Study the drawing (mm; zero at the part's minimum x, y, z) and answer. A direction names the side the tool comes from. Coordinates: 2 decimals unless noted, no trailing zeros. Order: outer loops, then holes, each group sorted by start corner. A loop starts at its lowest first (then second) coordinate and runs counter-clockwise, first axis right, second up. Notation, with made-up numbers: (18.25, 50.5) -> (68.25, 50.5) arc R32 cw to (68.25, 79.5) -> close; hole circle Ø8 at (29, -33.75). An arc over 180 degrees is marked (long way). Answer as CSV lines item,"result". Start each with the question number.
Item 1: Each of these flat-tipped pins is pushed along its axis until it touches: pin 1 Ø1.5 at (y, z) = (3.5, 1) entering from +X; pin 2 Ø2 at (x, z) = (10, 2) entering from +Y. Where does it stop, or does it pass through?
Item 2: Which of the six approach directions +Z, -Z, +X, -X, +Y, -Y give full straight-line access (tool end or side, diameter ignored) to the marked faces 4, 5 and 6?
Item 3: Section B-B (z = 4) is taken. Write down the section's boundary in (x, y), then the cut area to 3 significant figures.
Item 4: For a pull along Y with two mould halves and no side action, classify the marked faces 1, 2 and 3 as pulls with the +Y half, pulls with the -Y half, needs draft (parallel to the pull), parting line crosses it, or undercut.
Item 5: Section A-A (x = 16.3) is taken. Write down the section's boundary in (y, z), then the cut area to 3 significant figures.
Item 6: Straight lines are drawn through the part: L1, parallel to Y at x = 6.3, z = 5; L2, parallel to Z at x = 12, y = 2; L3, parallel to X at y = 6, z = 2.5. For each, find the intervals that lie inside material, in ascending order.
Item 7: Section D-D (z = 7.5) is taken. Write down the section's boundary in (x, y).
Item 8: Section C-C (x = 10.5) is taken. Write down the section's boundary in (y, z), then the cut area to 4 significant figures.
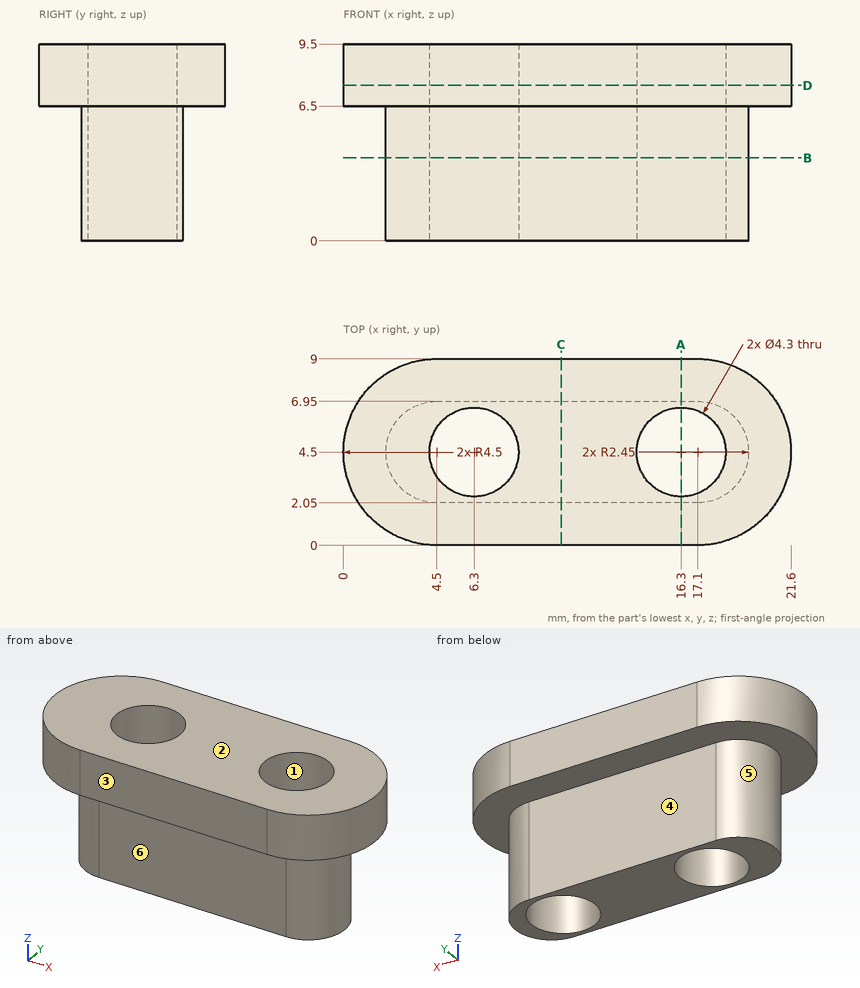
Checked values:
1,pin 1,"stops at x = 19.54"
1,pin 2,"stops at y = 6.95"
2,face 4,"-Z, +X, -X, +Y"
2,face 5,"-Z, -X"
2,face 6,"-Z, +X, -X, -Y"
3,outline,"(4.5, 2.05) -> (17.1, 2.05) arc R2.45 ccw to (17.1, 6.95) -> (4.5, 6.95) arc R2.45 ccw to start; hole circle Ø4.3 at (6.3, 4.5); hole circle Ø4.3 at (16.3, 4.5)"
3,area,"51.6 mm^2"
4,face 1,"undercut"
4,face 2,"needs draft"
4,face 3,"pulls with the -Y half"
5,outline,"(0, 6.5) -> (2.05, 6.5) -> (2.05, 0) -> (2.35, 0) -> (2.35, 9.5) -> (0, 9.5) -> close; (6.65, 0) -> (6.95, 0) -> (6.95, 6.5) -> (9, 6.5) -> (9, 9.5) -> (6.65, 9.5) -> close"
5,area,"18.0 mm^2"
6,L1,"y = 2.05 to 2.35, 6.65 to 6.95"
6,L2,"z = 6.5 to 9.5"
6,L3,"x = 2.56 to 4.76, 7.84 to 14.76, 17.84 to 19.04"
7,outline,"(4.5, 0) -> (17.1, 0) arc R4.5 ccw to (17.1, 9) -> (4.5, 9) arc R4.5 ccw to start; hole circle Ø4.3 at (6.3, 4.5); hole circle Ø4.3 at (16.3, 4.5)"
8,outline,"(0, 6.5) -> (2.05, 6.5) -> (2.05, 0) -> (6.95, 0) -> (6.95, 6.5) -> (9, 6.5) -> (9, 9.5) -> (0, 9.5) -> close"
8,area,"58.85 mm^2"
